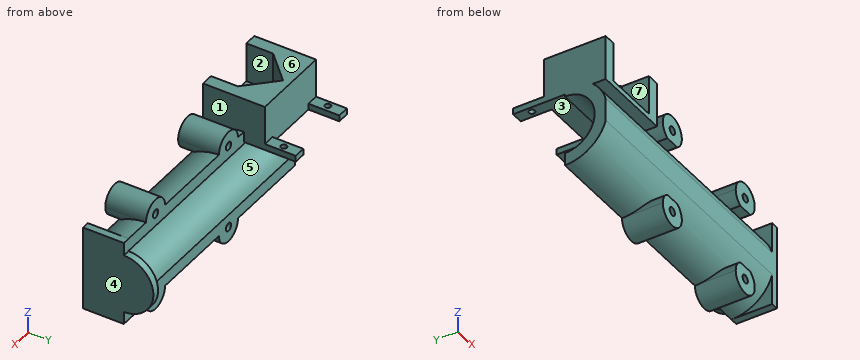
from build123d import *

# Parameters (mm, degrees)
SKETCH1_R           = 1.2
BOSS_EXTRUDE1_DEPTH = 2.5
SKETCH2_W           = 32.3
SKETCH2_H           = 25
BOSS_EXTRUDE2_DEPTH = 15.7
BOSS_EXTRUDE3_DEPTH = 105
BOSS_EXTRUDE4_START = 105
BOSS_EXTRUDE4_DEPTH = 3
BOSS_EXTRUDE5_DEPTH = 16.502469
SKETCH8_R           = 1.65
CUT_EXTRUDE1_DEPTH  = 46.267987394
CUT_EXTRUDE2_START  = 11
CUT_EXTRUDE2_DEPTH  = 2.6
CUT_EXTRUDE3_DEPTH  = 16


with BuildPart() as part:
    # Sketch1 → Boss-Extrude1 (new body)
    with BuildSketch(Plane.XY):
        Polygon((0, 0), (0, 37.5), (4.8, 37.5), (4.8, 25), (27.5, 25), (27.5, 37.5), (32.3, 37.5), (32.3, 0), align=None)
        with Locations((2.25, 31.25)):
            Circle(SKETCH1_R, mode=Mode.SUBTRACT)
        with Locations((30.05, 31.25)):
            Circle(SKETCH1_R, mode=Mode.SUBTRACT)
    extrude(amount=BOSS_EXTRUDE1_DEPTH)

    # Sketch2 → Boss-Extrude2 (add)
    with BuildSketch(Plane.XY.offset(2.5)):
        with Locations((16.15, 12.5)):
            Rectangle(SKETCH2_W, SKETCH2_H)
    extrude(amount=BOSS_EXTRUDE2_DEPTH)

    # Sketch4 → Boss-Extrude3 (add)
    with BuildSketch(Plane(origin=(0, 0, 0), x_dir=(0, 0, -1), z_dir=(1, 0, 0))):
        with BuildLine():
            ThreePointArc((-4.272382365, 16.502469348), (-0.788451938, 6.145596051), (8.24671518, 0))
            Line((8.24671518, 0), (17.480902455, 0))
            ThreePointArc((17.480902455, 0), (26.516069574, 6.145596051), (30, 16.502469348))
            Line((30, 16.502469348), (24.863808818, 16.502469348))
            ThreePointArc((24.863808818, 16.502469348), (12.863808818, 4.502469348), (0.863808818, 16.502469348))
            Line((0.863808818, 16.502469348), (-4.272382365, 16.502469348))
        make_face()
    extrude(amount=BOSS_EXTRUDE3_DEPTH)

    # Sketch5 → Boss-Extrude4 (add)
    with BuildSketch(Plane(origin=(0, 0, 0), x_dir=(0, 0, -1), z_dir=(1, 0, 0)).offset(BOSS_EXTRUDE4_START)):
        with BuildLine():
            Line((24.863808818, 16.502469348), (30, 16.502469348))
            Line((30, 16.502469348), (30, 0))
            Line((30, 0), (-4.276191182, 0))
            Line((-4.276191182, 0), (-4.276191182, 16.502469348))
            Line((-4.276191182, 16.502469348), (0.988808818, 16.502469348))
            ThreePointArc((0.988808818, 16.502469348), (12.926308818, 28.439969348), (24.863808818, 16.502469348))
        make_face()
    extrude(amount=BOSS_EXTRUDE4_DEPTH)

    # Sketch6 → Boss-Extrude5 (add)
    with BuildSketch(Plane(origin=(0, 16.502469348, 0), x_dir=(1, 0, 0), z_dir=(0, 1, 0))):
        with BuildLine():
            ThreePointArc((48, 30), (42, 36), (36, 30))
            Line((36, 30), (48, 30))
        make_face()
        with BuildLine():
            ThreePointArc((36, 30), (36.774618191, 27.051206187), (38.89846165, 24.863808818))
            Line((38.89846165, 24.863808818), (45.10153835, 24.863808818))
            ThreePointArc((45.10153835, 24.863808818), (47.225381809, 27.051206187), (48, 30))
            Line((48, 30), (36, 30))
        make_face()
        with BuildLine():
            ThreePointArc((45.098382452, 0.863808818), (47.224007714, -1.323058877), (48, -4.272382365))
            ThreePointArc((48, -4.272382365), (42.001904409, -10.272382062), (36.000001209, -4.276191181))
            ThreePointArc((36.000001209, -4.276191181), (36.775057034, -1.324717133), (38.901618757, 0.863808818))
            Line((38.901618757, 0.863808818), (45.098382452, 0.863808818))
        make_face()
        with BuildLine():
            ThreePointArc((91.095222125, 0.863808818), (93.223568356, -1.324186164), (94, -4.276191182))
            ThreePointArc((94, -4.276191182), (88, -10.276191182), (82, -4.276191182))
            ThreePointArc((82, -4.276191182), (82.776431644, -1.324186164), (84.904777875, 0.863808818))
            Line((84.904777875, 0.863808818), (91.095222125, 0.863808818))
        make_face()
        with BuildLine():
            ThreePointArc((94, 30), (88, 36), (82, 30))
            Line((82, 30), (94, 30))
        make_face()
        with BuildLine():
            ThreePointArc((82, 30), (82.774618191, 27.051206187), (84.89846165, 24.863808818))
            Line((84.89846165, 24.863808818), (91.10153835, 24.863808818))
            ThreePointArc((91.10153835, 24.863808818), (93.225381809, 27.051206187), (94, 30))
            Line((94, 30), (82, 30))
        make_face()
    extrude(amount=-BOSS_EXTRUDE5_DEPTH)

    # Sketch8 → Cut-Extrude1 (cut, through all)
    with BuildSketch(Plane(origin=(19.547405665, 45.267987294, 23.856702342), x_dir=(-1, 0, 0), z_dir=(0, 1, 0))):
        with Locations((-68.452594335, -19.58051116)):
            Circle(SKETCH8_R)
        with Locations((-22.452594335, -19.584319977)):
            Circle(SKETCH8_R)
        with Locations((-22.452594335, -53.856702342)):
            Circle(SKETCH8_R)
        with Locations((-68.452594335, -53.856702342)):
            Circle(SKETCH8_R)
    extrude(amount=-CUT_EXTRUDE1_DEPTH, mode=Mode.SUBTRACT)

    # Sketch9 → Cut-Extrude2 (cut)
    with BuildSketch(Plane(origin=(0, 0, 0), x_dir=(1, 0, 0), z_dir=(0, 1, 0)).offset(CUT_EXTRUDE2_START)):
        Polygon((45.348631561, 30), (43.674315781, 32.9), (40.325684219, 32.9), (38.651368439, 30), (40.325684219, 27.1), (43.674315781, 27.1), align=None)
        Polygon((91.348631561, 30), (89.674315781, 32.9), (86.325684219, 32.9), (84.651368439, 30), (86.325684219, 27.1), (89.674315781, 27.1), align=None)
        Polygon((45.348629319, -4.276258001), (43.677671059, -1.374322125), (40.32904174, -1.370446489), (38.651370681, -4.268506728), (40.322328941, -7.170442604), (43.67095826, -7.17431824), align=None)
        Polygon((91.348631561, -4.276191182), (89.674315781, -1.376191182), (86.325684219, -1.376191182), (84.651368439, -4.276191182), (86.325684219, -7.176191182), (89.674315781, -7.176191182), align=None)
    extrude(amount=CUT_EXTRUDE2_DEPTH, mode=Mode.SUBTRACT)

    # Sketch10 → Cut-Extrude3 (cut)
    with BuildSketch(Plane.XY.offset(18.2)):
        Polygon((5, 0), (27.3, 0), (27.3, 10.85), (16.15, 22), (5, 10.85), align=None)
    extrude(amount=-CUT_EXTRUDE3_DEPTH, mode=Mode.SUBTRACT)


solid = part.part
Work out the finished part from the listing and answer in its coordinate system (mm). Face numbers are marked on the shaded views. A direction names the side the tool comes from. Coordinates: 2 decimals unless noted, no trailing zeros. Order: outer loops, then holes, each group sorted by start corner. A loop starts at its lowest first (then second) coordinate and runs counter-clockwise, first axis right, second up. Notation, with made-up numbers: (9, -24.75) - (18, -24.75) arc R21 cw to (18, -4.75) - close; hole circle Ø6 at (79, -15). An arc over 180 degrees is marked (long way). Put each result on its own line as item: value. Start each with the question number.
1) Find section B-B (y = 31.25). Give the vertices of the cut face in (x, z).
2) Find section D-D (x = 88). State how many separate pieces and enclosed holes the cut face has, plus the area to 3 significant figures.
3) Flat-ended cylindrical pins translate along their axes: pin 1 (3.5 mm diameter, centred on x = 40.5, y = 2.5, fed in from +Z); pin 2 (1.7 mm diameter, centred on x = 40.5, z = -29, fed in from +Y); pin 3 (1 mm diameter, centred on x = 30, y = 26, fed in from +Z). Find the tip coordinate at first contact, or state that the pin passes through.
4) For the marked faces 5, 6 and 7, determine the directions among +Z, -Z, +X, -X, +Y, -Y from which every point of the face is accessible in a straight line to the end or side of a thin tool.
5) Find section C-C (y = 19). Give the vertices of the cut face in (x, z), plus the area to 3 significant figures.
6) For a pull along X with two mould halves and no side action, classify the marked faces 1, 2, 3 and 4 as released by +X, released by -X, zero draft, split by the parting line, or undercut.
7) Find section A-A (x = 30.05). Give the vertices of the cut face in (y, z).
8) Find the intervals of material crossed by line 1 (Y direction, x = 2.25, z = 0.65); line 2 (X direction, y = 31, z = 1); line 3 (Z direction, x = 88, y = 14.7), in increasing order. Write a range as from..to.
Results list:
1. outline: (0, 0) - (1.05, 0) - (1.05, 2.5) - (0, 2.5) - close; (3.45, 0) - (4.8, 0) - (4.8, 2.5) - (3.45, 2.5) - close; (27.5, 0) - (28.85, 0) - (28.85, 2.5) - (27.5, 2.5) - close; (31.25, 0) - (32.3, 0) - (32.3, 2.5) - (31.25, 2.5) - close
2. separate pieces: 3
2. enclosed holes: 0
2. area: 390 mm^2
3. pin 1: stops at z = 10.27
3. pin 2: stops at y = 16.5
3. pin 3: stops at z = 2.5
4. face 5: -X, +Y
4. face 6: +Z, +X, -X, +Y, -Y
4. face 7: +Z, -Y
5. outline: (0, 0) - (32.3, 0) - (32.3, 18.2) - (19.15, 18.2) - (19.15, 2.2) - (13.15, 2.2) - (13.15, 18.2) - (0, 18.2) - close; (105, -24.6) - (108, -24.6) - (108, -1.25) - (105, -1.25) - close
5. area: 562 mm^2
6. face 1: undercut
6. face 2: undercut
6. face 3: zero draft
6. face 4: released by +X
7. outline: (0, -17.48) arc R17.14 ccw to (16.5, -30) - (16.5, -24.86) arc R12 cw to (16.5, -0.86) - (16.5, 0) - (30.05, 0) - (30.05, 2.5) - (25, 2.5) - (25, 18.2) - (0, 18.2) - (0, 0) - (5.18, 0) arc R17.14 ccw to (0, -8.25) - close; (32.45, 0) - (37.5, 0) - (37.5, 2.5) - (32.45, 2.5) - close
8. line 1: y = 0..30.05, 32.45..37.5
8. line 2: x = 0..1.08, 3.42..4.8, 27.5..28.88, 31.22..32.3
8. line 3: z = -36..-31.65, -28.35..-24.73, -1..2.63, 5.93..10.28
